Design review of the part built by this model. Coordinates are the model's own, in mm. Face numbers are marked on the shaded views. A direction names the side the tool comes from. Give positions to 0.01 mm unless a question says otherwise; leave off trailing zeros. Order: outer loops, then holes, each group sorted by start corner. A loop starts at its lowest first (then second) coordinate and runs counter-clockwise, first axis right, second up. Notation, with made-up numbers: (84, 6.5) -> (120, 6.5) arc R23 cw to (120, 31.5) -> close; hole circle Ø7 at (31, 10.5). An arc over 180 degrees is marked (long way). One line per item, written item: value.
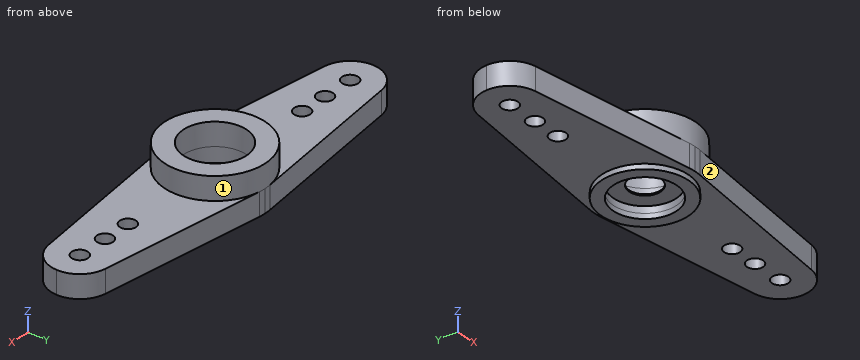
from build123d import *

# Parameters (mm, degrees)
F0_R     = 17.78
F1_DEPTH = 50.8
F2_R     = 111.76
F2_R_2   = 69.85
F3_DEPTH = 50.8
F4_R     = 69.85
F5_DEPTH = 83.82
F6_R     = 96.139
F6_R_2   = 69.85
F7_DEPTH = 11.43
F8_R     = 69.85
F9_DEPTH = 26.162


with BuildPart() as f1:
    # F0 (on Top) → F1 (new body)
    with BuildSketch(Plane.XY):
        with BuildLine():
            Line((223.52, 0), (34.925, 0))
            ThreePointArc((34.925, 0), (-24.695704, -24.695704), (0, 34.925))
            Line((0, 34.925), (0, 111.76))
            ThreePointArc((0, 111.76), (-7.141761, 111.531578), (-14.254328, 110.847245))
            Line((-14.254328, 110.847245), (-382.559843, 63.48524))
            ThreePointArc((-382.559843, 63.48524), (-422.45625, 42.275719), (-438.404, 0))
            ThreePointArc((-438.404, 0), (-422.45625, -42.275719), (-382.559843, -63.48524))
            Line((-382.559843, -63.48524), (-14.254328, -110.847245))
            ThreePointArc((-14.254328, -110.847245), (-7.141761, -111.531578), (0, -111.76))
            ThreePointArc((0, -111.76), (7.141761, -111.531578), (14.254328, -110.847245))
            Line((14.254328, -110.847245), (382.559843, -63.48524))
            ThreePointArc((382.559843, -63.48524), (422.45625, -42.275719), (438.404, 0))
            Line((438.404, 0), (392.176, 0))
            ThreePointArc((392.176, 0), (374.396, -17.78), (356.616, 0))
            Line((356.616, 0), (322.58, 0))
            ThreePointArc((322.58, 0), (304.8, -17.78), (287.02, 0))
            Line((287.02, 0), (259.08, 0))
            ThreePointArc((259.08, 0), (241.3, -17.78), (223.52, 0))
        make_face()
        with Locations((-374.396, 0)):
            Circle(F0_R, mode=Mode.SUBTRACT)
        with Locations((-304.8, 0)):
            Circle(F0_R, mode=Mode.SUBTRACT)
        with Locations((-241.3, 0)):
            Circle(F0_R, mode=Mode.SUBTRACT)
        with BuildLine():
            ThreePointArc((0, 34.925), (24.695704, 24.695704), (34.925, 0))
            Line((34.925, 0), (223.52, 0))
            ThreePointArc((223.52, 0), (241.3, 17.78), (259.08, 0))
            Line((259.08, 0), (287.02, 0))
            ThreePointArc((287.02, 0), (304.8, 17.78), (322.58, 0))
            Line((322.58, 0), (356.616, 0))
            ThreePointArc((356.616, 0), (374.396, 17.78), (392.176, 0))
            Line((392.176, 0), (438.404, 0))
            ThreePointArc((438.404, 0), (422.45625, 42.275719), (382.559843, 63.48524))
            Line((382.559843, 63.48524), (14.254328, 110.847245))
            ThreePointArc((14.254328, 110.847245), (7.141761, 111.531578), (0, 111.76))
            Line((0, 111.76), (0, 34.925))
        make_face()
    extrude(amount=F1_DEPTH)

    # F2 (on face) → F3 (join)
    with BuildSketch(Plane.XY.offset(50.8)):
        Circle(F2_R)
        Circle(F2_R_2, mode=Mode.SUBTRACT)
    extrude(amount=F3_DEPTH)

    # F4 (on face) → F5 (cut)
    with BuildSketch(Plane.XY.offset(101.6)):
        Circle(F4_R)
    extrude(amount=-F5_DEPTH, mode=Mode.SUBTRACT)

    # F6 (on face) → F7 (join)
    with BuildSketch(Plane(origin=(0, 0, 0), x_dir=(1, 0, 0), z_dir=(0, 0, -1))):
        Circle(F6_R)
        Circle(F6_R_2, mode=Mode.SUBTRACT)
    extrude(amount=F7_DEPTH)

    # F8 (on face) → F9 (cut)
    with BuildSketch(Plane(origin=(0, 0, -11.43), x_dir=(1, 0, 0), z_dir=(0, 0, -1))):
        Circle(F8_R)
    extrude(amount=-F9_DEPTH, mode=Mode.SUBTRACT)


solid = f1.part
Item 1: Machinability: for the marked faces 1 and 2, which of the approach directions +Z, -Z, +X, -X, +Y, -Y give a long, thin tool a straight path to every point of the face, cutting with its end or side? Answer none if there is none.
Returned:
face 1: +Z
face 2: +Z, -Z, +X, -Y
Item 2: Add section A-A on x = -302. Give the boundary of the cut face in (y, z), plus the area to 3 significant figures.
Returned:
outline: (-73.84, 0) -> (-17.56, 0) -> (-17.56, 50.8) -> (-73.84, 50.8) -> close; (17.56, 0) -> (73.84, 0) -> (73.84, 50.8) -> (17.56, 50.8) -> close
area: 5,720 mm²
Item 3: Add section C-C on y = -47.5. Give the boundary of the cut face in (x, z), plus the area to 3 significant figures.
Returned:
outline: (-417.3, 0) -> (-83.59, 0) -> (-83.59, -11.43) -> (-51.21, -11.43) -> (-51.21, 14.73) -> (51.21, 14.73) -> (51.21, -11.43) -> (83.59, -11.43) -> (83.59, 0) -> (417.3, 0) -> (417.3, 50.8) -> (101.16, 50.8) -> (101.16, 101.6) -> (51.21, 101.6) -> (51.21, 17.78) -> (-51.21, 17.78) -> (-51.21, 101.6) -> (-101.16, 101.6) -> (-101.16, 50.8) -> (-417.3, 50.8) -> close
area: 43,300 mm²
Item 4: Add section D-D on x = 304.8. Give the boundary of the cut face in (y, z).
Returned:
outline: (-73.48, 0) -> (-17.78, 0) -> (-17.78, 50.8) -> (-73.48, 50.8) -> close; (17.78, 0) -> (73.48, 0) -> (73.48, 50.8) -> (17.78, 50.8) -> close
Item 5: To check wall thickness, follow line 1 along X through (y, z) = (0, -6); line 2 along Y through (x, z) = (0, 91.5). State the ranges of each line that lie inside material, in increasing order. Write a range as from..to.
Returned:
line 1: -96.14..-69.85, 69.85..96.14
line 2: -111.76..-69.85, 69.85..111.76
Item 6: Clearance check with flat-ended pins moving along their axes: P1, Ø1, axis at x = -151.5, z = 23, coming from the +Y side; P2, Ø4, axis at x = -261, z = 49, coming from the -Y side; P3, Ø8, axis at x = -128, z = 40.5, coming from the +Y side. State where each tip first meets the part, or that it passes through.
Returned:
P1: y = 93.26
P2: y = -79.37
P3: y = 96.73
Item 7: Add section B-B on z = 70.5. Give the boundary of the cut face in (x, y).
Returned:
outline: circle Ø223.52 at (0, 0); hole circle Ø139.7 at (0, 0)
